from build123d import *

# Parameters (mm, degrees)
F1_R     = 29
F1_R_2   = 28.5
F2_DEPTH = 15
F3_W     = 7.017247
F3_H     = 1
F3_W_2   = 2
F3_H_2   = 7.017247
F4_DEPTH = 2
F5_R     = 5
F5_R_2   = 4.25
F6_DEPTH = 10


with BuildPart() as f2:
    # F1 (on Top) → F2 (new body)
    with BuildSketch(Plane.XY):
        with Locations((-36, 36)):
            Circle(F1_R)
        with Locations((-36, 36)):
            Circle(F1_R_2, mode=Mode.SUBTRACT)
    extrude(amount=F2_DEPTH)

    # F3 (on Top) → F4 (join)
    with BuildSketch(Plane.XY):
        Polygon((-16.377787, 14.963573), (-15.67068, 15.67068), (-36, 36), (-34.585786, 36), (-35.292893, 36.707107), (-55.622213, 57.036427), (-57.036427, 55.622213), (-36.707107, 35.292893), align=None)
        Polygon((-36, 36), (-15.67068, 15.67068), (-14.963573, 16.377787), (-34.585786, 36), align=None)
        with Locations((-3.508623, 36.5)):
            Rectangle(F3_W, F3_H)
        with Locations((-3.508623, 35.5)):
            Rectangle(F3_W, F3_H)
        with Locations((-36, 3.508623)):
            Rectangle(F3_W_2, F3_H_2)
        Polygon((-17.547779, 13.627795), (-17.547779, 0), (-15.547779, 0), (-15.547779, 15.440169), align=None)
        Polygon((0, 15.547779), (0, 17.547779), (-13.627795, 17.547779), (-15.440169, 15.547779), align=None)
    extrude(amount=F4_DEPTH)

    # F5 (on face) → F6 (join)
    with BuildSketch(Plane(origin=(0, 0, 0), x_dir=(1, 0, 0), z_dir=(0, 0, -1))):
        with Locations((-36, -36)):
            Circle(F5_R)
        with Locations((-36, -36)):
            Circle(F5_R_2, mode=Mode.SUBTRACT)
    extrude(amount=-F6_DEPTH)

    # F8: F2 across plane


with BuildPart() as f2_1:
    add(f2.part)
    add(f2.part.mirror(Plane.XZ))

    # F9: F2 across plane


with BuildPart() as f2_2:
    add(f2_1.part)
    add(f2_1.part.mirror(Plane.YZ))


solid = f2_2.part
Build history of the part. All positions in model axes, mm. A direction names the side the tool comes from. Round coordinates to 2 decimals unless told otherwise and drop trailing zeros. Write each loop counter-clockwise with the first axis right and the second up, starting at its lowest first coordinate (ties: lowest second). Pieces come first, ordered by that corner, then holes. Notation, with made-up numbers: M 55,-15.5 L 112,-15.5 A21 ccw 112,19.5 Z; hole C 80.5,78.5 d6. An arc over 180 degrees is marked long. Answer as a JSON object with one key per item and string values. Group by question number.
(1) Mould opens along X. For faces 4 (the flat face through (36.748, -35.334, 0.986)), 5 (the flat face through (-14.7, 16.8, 15)) say: pulls with the +X half, pulls with the -X half, needs draft (parallel to the pull), parting line crosses it, or undercut.
(2) Cut at B-B (y = 51.5). Give the cut face in (x, z).
(3) Flat gauge pins, fed straight in: pin 1 (3 mm diameter, centred on x = 33.5, y = 34, fed in from +Z); pin 2 (5 mm diameter, centred on x = 14.5, z = 10, fed in from -Y); pin 3 (1 mm diameter, centred on y = -2, z = 0.5, fed in from -X); pin 4 (3 mm diameter, centred on y = -34.5, z = 3.5, fed in from +X). Where does each tip first touch, or does it go through?
(4) Cut at A-A (y = 9). Give the cut face in (x, z), and give its area (3 significant figures).
(5) Which spindle directions (+Z, -Z, +X, -X, +Y, -Y) get a long thin tool onto all of the face, cutting with end or side? Do faces 1 (the flat face through (48.626, 47.212, 0.986)), 2 (the flat face through (14.7, -16.8, 15)), 3 (the flat face through (-38, -40, 10)). Say none if no direction does.
(6) Drill centre lines: L1, parallel to Y at x = -36, z = 10.5; L2, parallel to Y at x = 55.5, z = 8.25. Where is each one in solid material? Low to high.
Responses:
{
 "1": {"face 4": "undercut", "face 5": "needs draft"},
 "2": {"outline": "M -60.51,0 L -59.92,0 L -59.92,15 L -60.51,15 Z; M -52.91,0 L -50.09,0 L -50.09,2 L -52.91,2 Z; M -12.08,0 L -11.49,0 L -11.49,15 L -12.08,15 Z; M 11.49,0 L 12.08,0 L 12.08,15 L 11.49,15 Z; M 50.09,0 L 52.91,0 L 52.91,2 L 50.09,2 Z; M 59.92,0 L 60.51,0 L 60.51,15 L 59.92,15 Z"},
 "3": {"pin 1": "stops at z = 10", "pin 2": "stops at y = -57.91", "pin 3": "stops at x = -37", "pin 4": "stops at x = 65"},
 "4": {"outline": "M -46.58,0 L -45.12,0 L -45.12,15 L -46.58,15 Z; M -26.88,0 L -25.42,0 L -25.42,15 L -26.88,15 Z; M -17.55,0 L -15.55,0 L -15.55,2 L -17.55,2 Z; M 15.55,0 L 17.55,0 L 17.55,2 L 15.55,2 Z; M 25.42,0 L 26.88,0 L 26.88,15 L 25.42,15 Z; M 45.12,0 L 46.58,0 L 46.58,15 L 45.12,15 Z", "area": "95.5 mm2"},
 "5": {"face 1": "+Z, -Z", "face 2": "+Z, +X, -X, +Y, -Y", "face 3": "+Z"},
 "6": {"L1": "y = -65 to -64.5, -7.5 to -7, 7 to 7.5, 64.5 to 65", "L2": "y = -57.47 to -56.78, -15.22 to -14.53, 14.53 to 15.22, 56.78 to 57.47"}
}
